from build123d import *

# Parameters (mm, degrees)
SKETCH1_R           = 1.5
BOSS_EXTRUDE1_DEPTH = 3
CUT_EXTRUDE1_START  = -3
CUT_EXTRUDE1_DEPTH  = 3


with BuildPart() as part:
    # Sketch1 → Boss-Extrude1 (new body)
    with BuildSketch(Plane(origin=(0, 0, 0), x_dir=(1, 0, 0), z_dir=(0, 1, 0))):
        with BuildLine():
            Line((-5.292925578, 53.73997524), (-4.508788455, 45.778497427))
            ThreePointArc((-4.508788455, 45.778497427), (-2.257113019, 45.944590985), (0, 46))
            ThreePointArc((0, 46), (32.526911935, 32.526911935), (46, 0))
            ThreePointArc((46, 0), (45.944590985, -2.257113019), (45.778497427, -4.508788455))
            Line((45.778497427, -4.508788455), (53.73997524, -5.292925578))
            ThreePointArc((53.73997524, -5.292925578), (53.934954635, -2.649654414), (54, 0))
            ThreePointArc((54, 0), (36.264183562, 40.011360769), (-5.292925578, 53.73997524))
        make_face()
        with Locations(Location((50, 0, 0), (0, 0, 270))):
            Circle(SKETCH1_R, mode=Mode.SUBTRACT)
        with Locations(Location((49.03926402, 9.754516101, 0), (0, 0, 270))):
            Circle(SKETCH1_R, mode=Mode.SUBTRACT)
        with Locations(Location((46.193976626, 19.134171618, 0), (0, 0, 270))):
            Circle(SKETCH1_R, mode=Mode.SUBTRACT)
        with Locations(Location((0, 50, 0), (0, 0, 270))):
            Circle(SKETCH1_R, mode=Mode.SUBTRACT)
        with Locations(Location((9.754516101, 49.03926402, 0), (0, 0, 270))):
            Circle(SKETCH1_R, mode=Mode.SUBTRACT)
        with Locations(Location((19.134171618, 46.193976626, 0), (0, 0, 270))):
            Circle(SKETCH1_R, mode=Mode.SUBTRACT)
        with Locations(Location((35.355339059, 35.355339059, 0), (0, 0, 270))):
            Circle(SKETCH1_R, mode=Mode.SUBTRACT)
        with Locations(Location((41.573480615, 27.778511651, 0), (0, 0, 270))):
            Circle(SKETCH1_R, mode=Mode.SUBTRACT)
        with Locations(Location((27.778511651, 41.573480615, 0), (0, 0, 270))):
            Circle(SKETCH1_R, mode=Mode.SUBTRACT)
    extrude(amount=BOSS_EXTRUDE1_DEPTH)

    # Sketch2 → Cut-Extrude1 (cut)
    with BuildSketch(Plane(origin=(0, 3, 0), x_dir=(1, 0, 0), z_dir=(0, 1, 0)).offset(CUT_EXTRUDE1_START)):
        with BuildLine():
            ThreePointArc((1e-08, 46), (-4, 50.000000016), (4.3e-08, 54))
            ThreePointArc((4.3e-08, 54), (-2.649654392, 53.934954636), (-5.292925578, 53.73997524))
            Line((-5.292925578, 53.73997524), (-4.508788455, 45.778497427))
            ThreePointArc((-4.508788455, 45.778497427), (-2.257113014, 45.944590986), (1e-08, 46))
        make_face()
        with BuildLine():
            ThreePointArc((53.73997524, -5.292925578), (53.934954635, -2.649654414), (54, 0))
            ThreePointArc((54, 0), (49.999999885, -4), (46, 2.31e-07))
            ThreePointArc((46, 2.31e-07), (45.944590991, -2.257112904), (45.778497427, -4.508788455))
            Line((45.778497427, -4.508788455), (53.73997524, -5.292925578))
        make_face()
    extrude(amount=CUT_EXTRUDE1_DEPTH, mode=Mode.SUBTRACT)


solid = part.part
Verification items for the finished model (mm, model axes). Coordinates: 2 decimals unless noted, no trailing zeros. Order: outer loops, then holes, each group sorted by start corner. A loop starts at its lowest first (then second) coordinate and runs counter-clockwise, first axis right, second up. Notation, with made-up numbers: M -24,68.25 L -18,68.25 A27 ccw -18,102.25 Z; hole C 47,31 d10. An arc over 180 degrees is marked long. One line per item, written item: value. Start each with the question number.
Item 1: Scan lines: probe 1 along X at (y, z) = (1.65, -50); probe 2 along X at (y, z) = (0.9, -34.5); probe 3 along X at (y, z) = (1.6, -10.5). Record each from-to range of solid material in increasing order.
Item 2: Sectioned sample at A-A (y = 1.9). Count the separate pieces of the cut face and the enclosed holes in it, then the cut area to 3 significant figures.
Item 3: Mould release check, pull along X, two halves, no side actions. Record for faces 1 (the cylindrical face through (50, 1, 4)), 2 (the cylindrical face through (32.17, 1.48, -32.88)), 3 (the cylindrical face through (34.443, 1.479, -36.546)): released by +X, released by -X, zero draft, split by the parting line, or undercut.
Item 4: Sectioned sample at B-B (z = -3). Enter the section's corners in (x, y), then the cut area to 3 significant figures.
Item 5: Sectioned sample at C-C (x = 4). Enter the section's corners in (y, z).
Conclusion:
1. probe 1: x = -4 to -1.5, 1.5 to 8.6, 10.91 to 20.4
1. probe 2: x = 30.43 to 34.12, 36.59 to 41.54
1. probe 3: x = 44.79 to 47.74, 50.34 to 52.97
2. separate pieces: 1
2. enclosed holes: 9
2. area: 615 mm^2
3. face 1: split by the parting line
3. face 2: released by -X
3. face 3: undercut
4. outline: M 45.9,0 L 53.92,0 L 53.92,3 L 45.9,3 Z
4. area: 24.0 mm^2
5. outline: M 0,-53.85 L 3,-53.85 L 3,-45.83 L 0,-45.83 Z
